Design review of the part built by this model. Coordinates are the model's own, in mm. A direction names the side the tool comes from. Give positions to 0.01 mm unless a question says otherwise; leave off trailing zeros. Loops run counter-clockwise (first coordinate to the right, second up) from the corner with the lowest first, then second, coordinate; pieces in that order, holes last. Notation, with made-up numbers: M 65,13.25 L 104,13.25 A36 cw 104,48.25 Z; hole C 68.5,17.5 d7. An arc over 180 degrees is marked long. Use a Markdown table: item, result. Add a question column.
(1) Insertion check: pin 1 Ø7.5 at (x, z) = (99.5, -9.5) entering from +Y; pin 2 Ø2.5 at (x, y) = (-75, 12.5) entering from +Z; pin 3 Ø2 at (y, z) = (27, -18) entering from +X. Each pin has a flat end and moves straight along its axis. Give the tip position at first contact, or say it passes through.
(2) Add section A-A, the plane z = -25. Give the boundary of the cut face in (x, y).
(3) Add section B-B, the plane y = 12.5. Give the boundary of the cut face in (x, z), then the cut area to 3 significant figures.
(4) Add section C-C, the plane x = 75. Give the boundary of the cut face in (y, z), then the cut area to 3 significant figures.
(5) For faces 1 (the face through (100, 2, -1)), 2 (the face through (-75, 3, -25)), 3 (the face through (-73.092, 13.101, 55.035)), list the 3-axis set-ups (+Z, -Z, +X, -X, +Y, -Y) from which the entire face can be reached by the end or side of a thin tool; tool diameter is ignored.
(6) Draft analysis for pull direction Z (two halves, no side actions). For faces 4 (the face through (-2, 15, 57.5)), 5 (the face through (76.908, 11.899, -54.965)), 6 (the face through (-75, 12, -52.5)), 7 (the face through (92.5, 16, 1)), state which applies: pulls with the +Z half, pulls with the -Z half, needs draft (parallel to the pull), parting line crosses it, or undercut.
(7) Add section D-D, the plane z = 47. Give the boundary of the cut face in (x, y), then the cut area to 3 significant figures.
(8) For probe 1 along X at (y, z) = (12.5, -53.75); probe 2 along X at (y, z) = (12.5, -56.1); probe 3 along Y at (x, z) = (-75, -55), list the stretches that pass through material, from the lowest coordinate up.
```python
from build123d import *

# Parameters (mm, degrees)
SKETCH1_W           = 215
SKETCH1_H           = 115
BOSS_EXTRUDE1_DEPTH = 30
SKETCH2_W           = 15
SKETCH2_H           = 111
CUT_EXTRUDE1_DEPTH  = 28
SKETCH3_R           = 2
CUT_EXTRUDE2_DEPTH  = 5
SKETCH4_R           = 2
CUT_EXTRUDE3_DEPTH  = 3
CUT_EXTRUDE4_START  = -5
SKETCH5_R           = 2
CUT_EXTRUDE4_DEPTH  = 5


with BuildPart() as part:
    # Sketch1 → Boss-Extrude1 (new body)
    with BuildSketch(Plane(origin=(0, 0, 0), x_dir=(1, 0, 0), z_dir=(0, 1, 0))):
        Rectangle(SKETCH1_W, SKETCH1_H)
    extrude(amount=BOSS_EXTRUDE1_DEPTH)

    # Sketch2 → Cut-Extrude1 (cut)
    with BuildSketch(Plane(origin=(0, 30, 0), x_dir=(1, 0, 0), z_dir=(0, 1, 0))):
        with Locations((100, 0)):
            Rectangle(SKETCH2_W, SKETCH2_H)
    extrude(amount=-CUT_EXTRUDE1_DEPTH, mode=Mode.SUBTRACT)

    # Sketch3 → Cut-Extrude2 (cut)
    with BuildSketch(Plane.XY.offset(57.5)):
        with Locations((75, 12.5)):
            Circle(SKETCH3_R)
        with Locations((-75, 12.5)):
            Circle(SKETCH3_R)
    extrude(amount=-CUT_EXTRUDE2_DEPTH, mode=Mode.SUBTRACT)

    # Sketch4 → Cut-Extrude3 (cut)
    with BuildSketch(Plane.XZ):
        with Locations(Location((75, -25, 0), (0, 0, 270))):
            Circle(SKETCH4_R)
        with Locations(Location((-75, -25, 0), (0, 0, 270))):
            Circle(SKETCH4_R)
        with Locations(Location((-75, 25, 0), (0, 0, 270))):
            Circle(SKETCH4_R)
        with Locations(Location((75, 25, 0), (0, 0, 270))):
            Circle(SKETCH4_R)
    extrude(amount=-CUT_EXTRUDE3_DEPTH, mode=Mode.SUBTRACT)

    # Sketch5 → Cut-Extrude4 (cut)
    with BuildSketch(Plane(origin=(0, 0, -57.5), x_dir=(-1, 0, 0), z_dir=(0, 0, -1)).offset(CUT_EXTRUDE4_START)):
        with Locations(Location((-75, 12.5, 0), (0, 0, 180))):
            Circle(SKETCH5_R)
        with Locations(Location((75, 12.5, 0), (0, 0, 180))):
            Circle(SKETCH5_R)
    extrude(amount=CUT_EXTRUDE4_DEPTH, mode=Mode.SUBTRACT)


solid = part.part
```
Established:
| question | item | result |
|---|---|---|
| 1 | pin 1 | y = 2 |
| 1 | pin 2 | z = 52.5 |
| 1 | pin 3 | x = 92.5 |
| 2 | outline | M -107.5,0 L -77,0 L -77,3 L -73,3 L -73,0 L 73,0 L 73,3 L 77,3 L 77,0 L 107.5,0 L 107.5,2 L 92.5,2 L 92.5,30 L -107.5,30 Z |
| 3 | outline | M -107.5,-57.5 L -77,-57.5 L -77,-52.5 L -73,-52.5 L -73,-57.5 L 73,-57.5 L 73,-52.5 L 77,-52.5 L 77,-57.5 L 107.5,-57.5 L 107.5,-55.5 L 92.5,-55.5 L 92.5,55.5 L 107.5,55.5 L 107.5,57.5 L 77,57.5 L 77,52.5 L 73,52.5 L 73,57.5 L -73,57.5 L -73,52.5 L -77,52.5 L -77,57.5 L -107.5,57.5 Z |
| 3 | area | 23,000 mm^2 |
| 4 | outline | M 0,-57.5 L 10.5,-57.5 L 10.5,-52.5 L 14.5,-52.5 L 14.5,-57.5 L 30,-57.5 L 30,57.5 L 14.5,57.5 L 14.5,52.5 L 10.5,52.5 L 10.5,57.5 L 0,57.5 L 0,27 L 3,27 L 3,23 L 0,23 L 0,-23 L 3,-23 L 3,-27 L 0,-27 Z |
| 4 | area | 3,390 mm^2 |
| 5 | face 1 | +X, +Y |
| 5 | face 2 | -Y |
| 5 | face 3 | +Z |
| 6 | face 4 | pulls with the +Z half |
| 6 | face 5 | needs draft |
| 6 | face 6 | pulls with the -Z half |
| 6 | face 7 | undercut |
| 7 | outline | M -107.5,0 L 107.5,0 L 107.5,2 L 92.5,2 L 92.5,30 L -107.5,30 Z |
| 7 | area | 6,030 mm^2 |
| 8 | probe 1 | -107.5 to -77, -73 to 73, 77 to 92.5 |
| 8 | probe 2 | -107.5 to -77, -73 to 73, 77 to 107.5 |
| 8 | probe 3 | 0 to 10.5, 14.5 to 30 |
